Verification items for the finished model (mm, model axes). A direction names the side the tool comes from. Round coordinates to 2 decimals unless told otherwise and drop trailing zeros. Order: outer loops, then holes, each group sorted by start corner. A loop starts at its lowest first (then second) coordinate and runs counter-clockwise, first axis right, second up. Notation, with made-up numbers: (53.25, 84.25) -> (61.25, 84.25) arc R18 cw to (61.25, 107.25) -> close; hole circle Ø5 at (65.5, 62). An arc over 180 degrees is marked (long way). Return JSON: item names as keys, results as strings. Group by question number.
Item 1: Draft check along Y on faces 3 (the flat face through (6, 50, 1)), 4 (the cylindrical face through (11.74, 12.33, 0.49)), 5 (the flat face through (11, 25, 2)). Enter one of: pulls with the +Y half, pulls with the -Y half, needs draft (parallel to the pull), parting line crosses it, or undercut.
Item 2: Sectioned sample at A-A on x = 12. Record the cut outline in (y, z) (3 decimals).
Item 3: Sectioned sample at B-B on z = 9. Record the cut outline in (x, y), plus the area to 3 significant figures.
Item 4: Scan lines: probe 1 along Y at (x, z) = (12, 0.3) (3 decimals); probe 2 along Z at (x, y) = (1.3, 7.5); probe 3 along Y at (x, z) = (11, 1). Record each from-to range of solid material in increasing order. Write a range as from..to.
Item 5: Depth check by flat-ended pin: pin 1 Ø6.5 at (x, y) = (12, 10.345) entering from +Z; pin 2 Ø2.5 at (y, z) = (42.5, 9) entering from +X; pin 3 Ø3 at (y, z) = (21, 11) entering from +X; pin 4 Ø5 at (x, y) = (12, 39.655) entering from +Z. Enter the tip coordinate at first touch or a pass-through.
Item 6: Sectioned sample at C-C on y = 27.5. Record the cut outline in (x, z), plus the area to 3 significant figures.
Item 7: Sectioned sample at D-D on z = 5. Record the cut outline in (x, y), plus the area to 3 significant figures.
Item 8: Access from +Z, -Z, +X, -X, +Y, -Y to the whole of each face (thin tool, end or side, straight path). Record for faces 1 (the flat face through (0, 25, 6)), 2 (the flat face through (2, 25, 7)).
```python
from build123d import *

# Parameters (mm, degrees)
SKETCH_W        = 20
SKETCH_H        = 50
SKETCH_R        = 2
PAD_DEPTH       = 2
SKETCH001_W     = 2
SKETCH001_H     = 50
PAD001_DEPTH    = 13
SKETCH002_R     = 1.5
POCKET_DEPTH    = 10
CHAMFER_SIZE    = 1
CHAMFER001_SIZE = 1


with BuildPart() as part:
    # Sketch → Pad (new body)
    with BuildSketch(Plane.XY):
        with Locations((10, 25)):
            Rectangle(SKETCH_W, SKETCH_H)
        with Locations((12, 39.655)):
            Circle(SKETCH_R, mode=Mode.SUBTRACT)
        with Locations((12, 10.345)):
            Circle(SKETCH_R, mode=Mode.SUBTRACT)
    extrude(amount=PAD_DEPTH)

    # Sketch001 → Pad001 (join)
    with BuildSketch(Plane.XY):
        with Locations((1, 25)):
            Rectangle(SKETCH001_W, SKETCH001_H)
    extrude(amount=PAD001_DEPTH)

    # Sketch002 (on Face10 of Pad001) → Pocket (cut)
    with BuildSketch(Plane.YZ.offset(2)):
        with Locations((7.5, 9)):
            Circle(SKETCH002_R)
        with Locations((42.5, 9)):
            Circle(SKETCH002_R)
    extrude(amount=-POCKET_DEPTH, mode=Mode.SUBTRACT)

    # Chamfer
    chamfer_edges = [part.edges().sort_by_distance(p)[0] for p in [
        (10, 39.655, 2),
        (10, 10.345, 2),
    ]]
    chamfer(chamfer_edges, length=CHAMFER_SIZE)

    # Chamfer001
    chamfer001_edges = [part.edges().sort_by_distance(p)[0] for p in [
        (0, 41, 9),
        (0, 6, 9),
    ]]
    chamfer(chamfer001_edges, length=CHAMFER001_SIZE)


solid = part.part
```
Recorded:
{
 "1": {"face 3": "pulls with the +Y half", "face 4": "undercut", "face 5": "needs draft"},
 "2": {"outline": "(0, 0) -> (8.345, 0) -> (8.345, 1) -> (7.345, 2) -> (0, 2) -> close; (12.345, 0) -> (37.655, 0) -> (37.655, 1) -> (36.655, 2) -> (13.345, 2) -> (12.345, 1) -> close; (41.655, 0) -> (50, 0) -> (50, 2) -> (42.655, 2) -> (41.655, 1) -> close"},
 "3": {"outline": "(0, 0) -> (2, 0) -> (2, 6) -> (1, 6) -> (0, 5) -> close; (0, 10) -> (1, 9) -> (2, 9) -> (2, 41) -> (1, 41) -> (0, 40) -> close; (0, 45) -> (1, 44) -> (2, 44) -> (2, 50) -> (0, 50) -> close", "area": "86.0 mm²"},
 "4": {"probe 1": "0..8.345, 12.345..37.655, 41.655..50", "probe 2": "0..7.5, 10.5..13", "probe 3": "0..8.61, 12.08..37.92, 41.39..50"},
 "5": {"pin 1": "z = 2", "pin 2": "through", "pin 3": "x = 2", "pin 4": "z = 1.5"},
 "6": {"outline": "(0, 0) -> (20, 0) -> (20, 2) -> (2, 2) -> (2, 13) -> (0, 13) -> close", "area": "62.0 mm²"},
 "7": {"outline": "(0, 0) -> (2, 0) -> (2, 50) -> (0, 50) -> close", "area": "100 mm²"},
 "8": {"face 1": "+Z, -Z, -X, +Y, -Y", "face 2": "+Z, +X, +Y, -Y"}
}
